Geometry check sheet. Reference: the model listing, model coordinates, mm. Round coordinates to 2 decimals unless told otherwise and drop trailing zeros. Use one line per item in the form item = value. Start each with the question number.
1. Cross-section at A-A (z = 2.05). State how many separate pieces and enclosed holes the cut face has, then the cut area to 3 significant figures.
2. Go/stop test with flat-tipped pins: pin 1 (4 mm diameter, centred on x = 58.3, y = -53.2, fed in from -Z); pin 2 (1.6 mm diameter, centred on x = -58.3, y = -60.2, fed in from -Z). Record where each tip stops, or that it passes through.
3. Material ranges on line 1 (X direction, y = 13, z = 0.65); line 2 (X direction, y = -24.5, z = 2.65); line 3 (Y direction, x = 60.5, z = 2.7), recorded low to high.
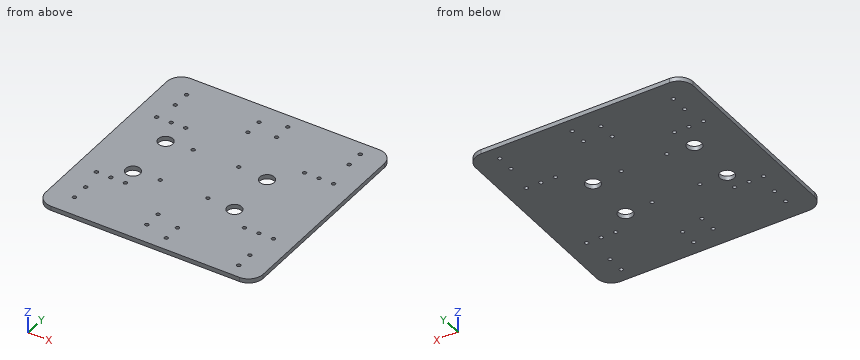
```python
from build123d import *

# Parameters (mm, degrees)
EXTRUDE_1_DEPTH     = 3
SKETCH_8_R          = 1.3
CUT_EXTRUDE_3_DEPTH = 3
CUT_EXTRUDE_7_REACH = 5
SKETCH_15_R         = 1.3
SKETCH_15_R_2       = 5


with BuildPart() as part:
    # 草图1 → 凸台-拉伸1 (new body)
    with BuildSketch(Plane.XY):
        with BuildLine():
            Line((-65, -75), (65, -75))
            ThreePointArc((65, -75), (72.071067812, -72.071067812), (75, -65))
            Line((75, -65), (75, 65))
            ThreePointArc((75, 65), (72.071067812, 72.071067812), (65, 75))
            Line((65, 75), (-65, 75))
            ThreePointArc((-65, 75), (-72.071067812, 72.071067812), (-75, 65))
            Line((-75, 65), (-75, -65))
            ThreePointArc((-75, -65), (-72.071067812, -72.071067812), (-65, -75))
        make_face()
    extrude(amount=EXTRUDE_1_DEPTH)

    # 草图8 → 切除-拉伸3 (cut)
    with BuildSketch(Plane(origin=(0, 0, 0), x_dir=(-1, 0, 0), z_dir=(0, 0, -1))):
        with Locations((8.299978541, 60.2)):
            Circle(SKETCH_8_R)
        with Locations((8.299978541, 48.2)):
            Circle(SKETCH_8_R)
        with Locations((8.299978541, -48.2)):
            Circle(SKETCH_8_R)
        with Locations((8.299978541, -60.2)):
            Circle(SKETCH_8_R)
        with Locations((58.299978541, -48.2)):
            Circle(SKETCH_8_R)
        with Locations((58.299978541, -60.2)):
            Circle(SKETCH_8_R)
        with Locations((58.299978541, 60.2)):
            Circle(SKETCH_8_R)
        with Locations((58.299978541, 48.2)):
            Circle(SKETCH_8_R)
        with Locations((-58.299978541, 65.2)):
            Circle(SKETCH_8_R)
        with Locations((-58.299978541, 53.2)):
            Circle(SKETCH_8_R)
        with Locations((-8.299978541, 53.2)):
            Circle(SKETCH_8_R)
        with Locations((-8.299978541, 65.2)):
            Circle(SKETCH_8_R)
        with Locations((-8.299978541, -65.2)):
            Circle(SKETCH_8_R)
        with Locations((-8.299978541, -53.2)):
            Circle(SKETCH_8_R)
        with Locations((-58.299978541, -53.2)):
            Circle(SKETCH_8_R)
        with Locations((-58.299978541, -65.2)):
            Circle(SKETCH_8_R)
    extrude(amount=-CUT_EXTRUDE_3_DEPTH, mode=Mode.SUBTRACT)

    # 草图15 → 切除-拉伸7 (cut, up to next)
    with BuildSketch(Plane(origin=(0, 0, 0), x_dir=(-1, 0, 0), z_dir=(0, 0, -1)), mode=Mode.PRIVATE) as cut_extrude_7_sk1:
        with Locations((-5.764701549, 16.542565405)):
            Circle(SKETCH_15_R)
    cut_extrude_7_tool1 = extrude(cut_extrude_7_sk1.sketch, amount=-CUT_EXTRUDE_7_REACH, mode=Mode.PRIVATE) & part.part
    add(cut_extrude_7_tool1.solids().sort_by_distance((5.764702, 16.542565, 0))[0], mode=Mode.SUBTRACT)
    # 草图15 → 切除-拉伸7 (cut, up to next)
    with BuildSketch(Plane(origin=(0, 0, 0), x_dir=(-1, 0, 0), z_dir=(0, 0, -1)), mode=Mode.PRIVATE) as cut_extrude_7_sk2:
        with Locations((25.680561341, 16.542565405)):
            Circle(SKETCH_15_R)
    cut_extrude_7_tool2 = extrude(cut_extrude_7_sk2.sketch, amount=-CUT_EXTRUDE_7_REACH, mode=Mode.PRIVATE) & part.part
    add(cut_extrude_7_tool2.solids().sort_by_distance((-25.680561, 16.542565, 0))[0], mode=Mode.SUBTRACT)
    # 草图15 → 切除-拉伸7 (cut, up to next)
    with BuildSketch(Plane(origin=(0, 0, 0), x_dir=(-1, 0, 0), z_dir=(0, 0, -1)), mode=Mode.PRIVATE) as cut_extrude_7_sk3:
        with Locations((25.680561341, -18.966705613)):
            Circle(SKETCH_15_R)
    cut_extrude_7_tool3 = extrude(cut_extrude_7_sk3.sketch, amount=-CUT_EXTRUDE_7_REACH, mode=Mode.PRIVATE) & part.part
    add(cut_extrude_7_tool3.solids().sort_by_distance((-25.680561, -18.966706, 0))[0], mode=Mode.SUBTRACT)
    # 草图15 → 切除-拉伸7 (cut, up to next)
    with BuildSketch(Plane(origin=(0, 0, 0), x_dir=(-1, 0, 0), z_dir=(0, 0, -1)), mode=Mode.PRIVATE) as cut_extrude_7_sk4:
        with Locations((-7.339504699, -18.966705613)):
            Circle(SKETCH_15_R)
    cut_extrude_7_tool4 = extrude(cut_extrude_7_sk4.sketch, amount=-CUT_EXTRUDE_7_REACH, mode=Mode.PRIVATE) & part.part
    add(cut_extrude_7_tool4.solids().sort_by_distance((7.339505, -18.966706, 0))[0], mode=Mode.SUBTRACT)
    # 草图15 → 切除-拉伸7 (cut, up to next)
    with BuildSketch(Plane(origin=(0, 0, 0), x_dir=(-1, 0, 0), z_dir=(0, 0, -1)), mode=Mode.PRIVATE) as cut_extrude_7_sk5:
        with Locations((43.674011713, 14.90502858)):
            Circle(SKETCH_15_R_2)
    cut_extrude_7_tool5 = extrude(cut_extrude_7_sk5.sketch, amount=-CUT_EXTRUDE_7_REACH, mode=Mode.PRIVATE) & part.part
    add(cut_extrude_7_tool5.solids().sort_by_distance((-43.674012, 14.905029, 0))[0], mode=Mode.SUBTRACT)
    # 草图15 → 切除-拉伸7 (cut, up to next)
    with BuildSketch(Plane(origin=(0, 0, 0), x_dir=(-1, 0, 0), z_dir=(0, 0, -1)), mode=Mode.PRIVATE) as cut_extrude_7_sk6:
        with Locations((43.674011713, -20.09497142)):
            Circle(SKETCH_15_R_2)
    cut_extrude_7_tool6 = extrude(cut_extrude_7_sk6.sketch, amount=-CUT_EXTRUDE_7_REACH, mode=Mode.PRIVATE) & part.part
    add(cut_extrude_7_tool6.solids().sort_by_distance((-43.674012, -20.094971, 0))[0], mode=Mode.SUBTRACT)
    # 草图15 → 切除-拉伸7 (cut, up to next)
    with BuildSketch(Plane(origin=(0, 0, 0), x_dir=(-1, 0, 0), z_dir=(0, 0, -1)), mode=Mode.PRIVATE) as cut_extrude_7_sk7:
        with Locations((-26.325988287, 14.90502858)):
            Circle(SKETCH_15_R_2)
    cut_extrude_7_tool7 = extrude(cut_extrude_7_sk7.sketch, amount=-CUT_EXTRUDE_7_REACH, mode=Mode.PRIVATE) & part.part
    add(cut_extrude_7_tool7.solids().sort_by_distance((26.325988, 14.905029, 0))[0], mode=Mode.SUBTRACT)
    # 草图15 → 切除-拉伸7 (cut, up to next)
    with BuildSketch(Plane(origin=(0, 0, 0), x_dir=(-1, 0, 0), z_dir=(0, 0, -1)), mode=Mode.PRIVATE) as cut_extrude_7_sk8:
        with Locations((-26.325988287, -20.09497142)):
            Circle(SKETCH_15_R_2)
    cut_extrude_7_tool8 = extrude(cut_extrude_7_sk8.sketch, amount=-CUT_EXTRUDE_7_REACH, mode=Mode.PRIVATE) & part.part
    add(cut_extrude_7_tool8.solids().sort_by_distance((26.325988, -20.094971, 0))[0], mode=Mode.SUBTRACT)
    # 草图15 → 切除-拉伸7 (cut, up to next)
    with BuildSketch(Plane(origin=(0, 0, 0), x_dir=(-1, 0, 0), z_dir=(0, 0, -1)), mode=Mode.PRIVATE) as cut_extrude_7_sk9:
        with Locations((-51.0383219, 32.287530058)):
            Circle(SKETCH_15_R)
    cut_extrude_7_tool9 = extrude(cut_extrude_7_sk9.sketch, amount=-CUT_EXTRUDE_7_REACH, mode=Mode.PRIVATE) & part.part
    add(cut_extrude_7_tool9.solids().sort_by_distance((51.038322, 32.28753, 0))[0], mode=Mode.SUBTRACT)
    # 草图15 → 切除-拉伸7 (cut, up to next)
    with BuildSketch(Plane(origin=(0, 0, 0), x_dir=(-1, 0, 0), z_dir=(0, 0, -1)), mode=Mode.PRIVATE) as cut_extrude_7_sk10:
        with Locations((51.0383219, 32.287530058)):
            Circle(SKETCH_15_R)
    cut_extrude_7_tool10 = extrude(cut_extrude_7_sk10.sketch, amount=-CUT_EXTRUDE_7_REACH, mode=Mode.PRIVATE) & part.part
    add(cut_extrude_7_tool10.solids().sort_by_distance((-51.038322, 32.28753, 0))[0], mode=Mode.SUBTRACT)
    # 草图15 → 切除-拉伸7 (cut, up to next)
    with BuildSketch(Plane(origin=(0, 0, 0), x_dir=(-1, 0, 0), z_dir=(0, 0, -1)), mode=Mode.PRIVATE) as cut_extrude_7_sk11:
        with Locations((51.0383219, -32.287530058)):
            Circle(SKETCH_15_R)
    cut_extrude_7_tool11 = extrude(cut_extrude_7_sk11.sketch, amount=-CUT_EXTRUDE_7_REACH, mode=Mode.PRIVATE) & part.part
    add(cut_extrude_7_tool11.solids().sort_by_distance((-51.038322, -32.28753, 0))[0], mode=Mode.SUBTRACT)
    # 草图15 → 切除-拉伸7 (cut, up to next)
    with BuildSketch(Plane(origin=(0, 0, 0), x_dir=(-1, 0, 0), z_dir=(0, 0, -1)), mode=Mode.PRIVATE) as cut_extrude_7_sk12:
        with Locations((-51.0383219, -32.287530058)):
            Circle(SKETCH_15_R)
    cut_extrude_7_tool12 = extrude(cut_extrude_7_sk12.sketch, amount=-CUT_EXTRUDE_7_REACH, mode=Mode.PRIVATE) & part.part
    add(cut_extrude_7_tool12.solids().sort_by_distance((51.038322, -32.28753, 0))[0], mode=Mode.SUBTRACT)
    # 草图15 → 切除-拉伸7 (cut, up to next)
    with BuildSketch(Plane(origin=(0, 0, 0), x_dir=(-1, 0, 0), z_dir=(0, 0, -1)), mode=Mode.PRIVATE) as cut_extrude_7_sk13:
        with Locations((-41.0383219, 32.287530058)):
            Circle(SKETCH_15_R)
    cut_extrude_7_tool13 = extrude(cut_extrude_7_sk13.sketch, amount=-CUT_EXTRUDE_7_REACH, mode=Mode.PRIVATE) & part.part
    add(cut_extrude_7_tool13.solids().sort_by_distance((41.038322, 32.28753, 0))[0], mode=Mode.SUBTRACT)
    # 草图15 → 切除-拉伸7 (cut, up to next)
    with BuildSketch(Plane(origin=(0, 0, 0), x_dir=(-1, 0, 0), z_dir=(0, 0, -1)), mode=Mode.PRIVATE) as cut_extrude_7_sk14:
        with Locations((61.0383219, 32.287530058)):
            Circle(SKETCH_15_R)
    cut_extrude_7_tool14 = extrude(cut_extrude_7_sk14.sketch, amount=-CUT_EXTRUDE_7_REACH, mode=Mode.PRIVATE) & part.part
    add(cut_extrude_7_tool14.solids().sort_by_distance((-61.038322, 32.28753, 0))[0], mode=Mode.SUBTRACT)
    # 草图15 → 切除-拉伸7 (cut, up to next)
    with BuildSketch(Plane(origin=(0, 0, 0), x_dir=(-1, 0, 0), z_dir=(0, 0, -1)), mode=Mode.PRIVATE) as cut_extrude_7_sk15:
        with Locations((61.0383219, -32.287530058)):
            Circle(SKETCH_15_R)
    cut_extrude_7_tool15 = extrude(cut_extrude_7_sk15.sketch, amount=-CUT_EXTRUDE_7_REACH, mode=Mode.PRIVATE) & part.part
    add(cut_extrude_7_tool15.solids().sort_by_distance((-61.038322, -32.28753, 0))[0], mode=Mode.SUBTRACT)
    # 草图15 → 切除-拉伸7 (cut, up to next)
    with BuildSketch(Plane(origin=(0, 0, 0), x_dir=(-1, 0, 0), z_dir=(0, 0, -1)), mode=Mode.PRIVATE) as cut_extrude_7_sk16:
        with Locations((-41.0383219, -32.287530058)):
            Circle(SKETCH_15_R)
    cut_extrude_7_tool16 = extrude(cut_extrude_7_sk16.sketch, amount=-CUT_EXTRUDE_7_REACH, mode=Mode.PRIVATE) & part.part
    add(cut_extrude_7_tool16.solids().sort_by_distance((41.038322, -32.28753, 0))[0], mode=Mode.SUBTRACT)
    # 草图15 → 切除-拉伸7 (cut, up to next)
    with BuildSketch(Plane(origin=(0, 0, 0), x_dir=(-1, 0, 0), z_dir=(0, 0, -1)), mode=Mode.PRIVATE) as cut_extrude_7_sk17:
        with Locations((-61.0383219, -32.287530058)):
            Circle(SKETCH_15_R)
    cut_extrude_7_tool17 = extrude(cut_extrude_7_sk17.sketch, amount=-CUT_EXTRUDE_7_REACH, mode=Mode.PRIVATE) & part.part
    add(cut_extrude_7_tool17.solids().sort_by_distance((61.038322, -32.28753, 0))[0], mode=Mode.SUBTRACT)
    # 草图15 → 切除-拉伸7 (cut, up to next)
    with BuildSketch(Plane(origin=(0, 0, 0), x_dir=(-1, 0, 0), z_dir=(0, 0, -1)), mode=Mode.PRIVATE) as cut_extrude_7_sk18:
        with Locations((41.0383219, -32.287530058)):
            Circle(SKETCH_15_R)
    cut_extrude_7_tool18 = extrude(cut_extrude_7_sk18.sketch, amount=-CUT_EXTRUDE_7_REACH, mode=Mode.PRIVATE) & part.part
    add(cut_extrude_7_tool18.solids().sort_by_distance((-41.038322, -32.28753, 0))[0], mode=Mode.SUBTRACT)
    # 草图15 → 切除-拉伸7 (cut, up to next)
    with BuildSketch(Plane(origin=(0, 0, 0), x_dir=(-1, 0, 0), z_dir=(0, 0, -1)), mode=Mode.PRIVATE) as cut_extrude_7_sk19:
        with Locations((41.0383219, 32.287530058)):
            Circle(SKETCH_15_R)
    cut_extrude_7_tool19 = extrude(cut_extrude_7_sk19.sketch, amount=-CUT_EXTRUDE_7_REACH, mode=Mode.PRIVATE) & part.part
    add(cut_extrude_7_tool19.solids().sort_by_distance((-41.038322, 32.28753, 0))[0], mode=Mode.SUBTRACT)
    # 草图15 → 切除-拉伸7 (cut, up to next)
    with BuildSketch(Plane(origin=(0, 0, 0), x_dir=(-1, 0, 0), z_dir=(0, 0, -1)), mode=Mode.PRIVATE) as cut_extrude_7_sk20:
        with Locations((-61.0383219, 32.287530058)):
            Circle(SKETCH_15_R)
    cut_extrude_7_tool20 = extrude(cut_extrude_7_sk20.sketch, amount=-CUT_EXTRUDE_7_REACH, mode=Mode.PRIVATE) & part.part
    add(cut_extrude_7_tool20.solids().sort_by_distance((61.038322, 32.28753, 0))[0], mode=Mode.SUBTRACT)


solid = part.part
```
Reported:
q1.separate_pieces = 1
q1.enclosed_holes = 36
q1.area = 21,900 mm²
q2.pin_1 = 0
q2.pin_2 = through
q3.line_1 = -75 to -48.3, -39.05 to 21.7, 30.95 to 75
q3.line_2 = -75 to -46.04, -41.31 to 23.96, 28.69 to 75
q3.line_3 = -75 to -33.47, -31.1 to 31.1, 33.47 to 75
